```python
from build123d import *

# Parameters (mm, degrees)
SKETCH1_W           = 45
SKETCH1_H           = 45
BOSS_EXTRUDE1_DEPTH = 300
SKETCH2_W           = 500
SKETCH2_H           = 45
BOSS_EXTRUDE2_DEPTH = 45
SHELL2_T            = -5
CUT_EXTRUDE1_DEPTH  = 45
SKETCH5_R           = 51.5
BOSS_EXTRUDE3_DEPTH = 2


with BuildPart() as part:
    # Sketch1 → Boss-Extrude1 (new body)
    with BuildSketch(Plane(origin=(0, 0, 0), x_dir=(1, 0, 0), z_dir=(0, 1, 0))):
        Rectangle(SKETCH1_W, SKETCH1_H)
    extrude(amount=BOSS_EXTRUDE1_DEPTH)

    # Sketch2 → Boss-Extrude2 (add)
    with BuildSketch(Plane(origin=(0, 300, 0), x_dir=(1, 0, 0), z_dir=(0, 1, 0))):
        Rectangle(SKETCH2_W, SKETCH2_H)
    extrude(amount=BOSS_EXTRUDE2_DEPTH)

    # Shell2
    shell2_openings = [part.faces().sort_by_distance(p)[0] for p in [
        (250, 322.5, 0),
        (-250, 322.5, 0),
        (0, 0, 0),
    ]]
    offset(amount=SHELL2_T, openings=shell2_openings, kind=Kind.INTERSECTION)

    # Sketch4 → Cut-Extrude1 (cut)
    with BuildSketch(Plane.XY.offset(22.5)):
        Polygon((-250, 300), (-172.057713659, 345), (-187.263807884, 591.817806189), (-292.402197695, 585.340379431), (-265.544239109, 495.362755895), align=None)
    cut_extrude1 = extrude(amount=-CUT_EXTRUDE1_DEPTH, mode=Mode.SUBTRACT)

    # Sketch5 → Boss-Extrude3 (add)
    with BuildSketch(Plane(origin=(-192.403810568, 333.253175473, 0), x_dir=(0.8660254037844376, 0.500000000000002, 0), z_dir=(-0.5000000000000019, 0.8660254037844375, 0))):
        with Locations(Location((-21.506350946, 0, 0), (0, 0, 180))):
            Circle(SKETCH5_R)
    boss_extrude3 = extrude(amount=BOSS_EXTRUDE3_DEPTH)

    # Mirror1: Cut-Extrude1, Boss-Extrude3 across plane
    add(cut_extrude1.mirror(Plane(origin=(0, 0, 0), x_dir=(0, 0, 1), z_dir=(1, 0, 0))), mode=Mode.SUBTRACT)
    add(boss_extrude3.mirror(Plane(origin=(0, 0, 0), x_dir=(0, 0, 1), z_dir=(1, 0, 0))))


solid = part.part
```
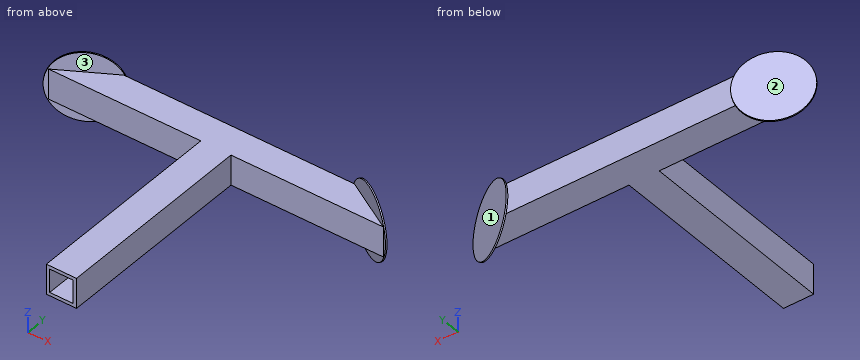
Source: CAD feature listing. Evaluate the final solid. Frame: model axes, mm. Face numbers are marked on the shaded views. Round coordinates to 2 decimals unless told otherwise and drop trailing zeros. Loops run counter-clockwise (first coordinate to the right, second up) from the corner with the lowest first, then second, coordinate; pieces in that order, holes last. Notation, with made-up numbers: (1.25, 63) - (22.25, 63) arc R28 ccw to (22.25, 90) - close; hole circle Ø1 at (-3, 63.5). An arc over 180 degrees is marked (long way). Use CSV: the item, a comma, the result in double quotes.
Q1. Mould query, pull axis X, two halves, no side actions, for the marked faces 1, 2 and 3. Classes: pulls with the +X half, pulls with the -X half, needs draft (parallel to the pull), parting line crosses it, or undercut.
Reported:
face 1,"pulls with the +X half"
face 2,"pulls with the -X half"
face 3,"undercut"
Q2. Section query A-A, the plane x = -81. Output: boundary loops of the cut face in (y, z).
Reported:
outline,"(300, -22.5) - (345, -22.5) - (345, 22.5) - (300, 22.5) - close; hole (305, -17.5) - (340, -17.5) - (340, 17.5) - (305, 17.5) - close"
Q3. Section query B-B, the plane z = 42.5. Output: boundary loops of the cut face in (x, y), then the cut area to 3 significant figures.
Reported:
outline,"(-237.22, 309.69) - (-236.22, 307.96) - (-185.84, 337.04) - (-186.84, 338.78) - close; (185.84, 337.04) - (236.22, 307.96) - (237.22, 309.69) - (186.84, 338.78) - close"
area,"233 mm^2"
Q4. Pin query (flat end, axial travel): pin 1 Ø17.5 at (x, z) = (116.5, -6.5) entering from +Y; pin 2 Ø13.5 at (y, z) = (207, -5.5) entering from -X; pin 3 Ø22.5 at (x, z) = (90, 10) entering from -Y. Return the tip coordinate at first contact, or that it passes through.
Reported:
pin 1,"y = 345"
pin 2,"x = -22.5"
pin 3,"y = 300"
Q5. Section query D-D, the plane z = -29. Output: boundary loops of the cut face in (x, y).
Reported:
outline,"(-248.89, 302.95) - (-247.89, 301.22) - (-174.17, 343.78) - (-175.17, 345.51) - close; (174.17, 343.78) - (247.89, 301.22) - (248.89, 302.95) - (175.17, 345.51) - close"
Q6. Ray query, line 1 along X through (y, z) = (42, 12); line 2 along Y through (x, z) = (-169.5, 2.5); line 3 along Y through (x, z) = (89.5, -0.5). Return the intervals inside material, ascending.
Reported:
line 1,"-22.5 to -17.5, 17.5 to 22.5"
line 2,"300 to 305, 340 to 345, 346.48 to 348.79"
line 3,"300 to 305, 340 to 345"
Q7. Section query C-C, the plane y = 96.5. Output: boundary loops of the cut face in (x, z).
Reported:
outline,"(-22.5, -22.5) - (22.5, -22.5) - (22.5, 22.5) - (-22.5, 22.5) - close; hole (-17.5, -17.5) - (17.5, -17.5) - (17.5, 17.5) - (-17.5, 17.5) - close"
